Part model, mm, in its own coordinate system. Face numbers are marked on the shaded views. A direction names the side the tool comes from. Coordinates: 2 decimals unless noted, no trailing zeros. Write each loop counter-clockwise with the first axis right and the second up, starting at its lowest first coordinate (ties: lowest second). Pieces come first, ordered by that corner, then holes. Notation, with made-up numbers: (25, -21.75) - (29, -21.75) arc R14 cw to (29, -17.75) - close; hole circle Ø11 at (37, 7). An arc over 180 degrees is marked (long way). Use a Markdown table: item, result.
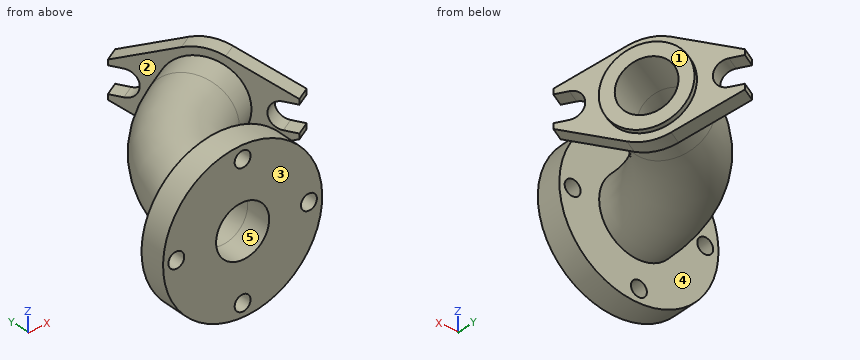
```python
from build123d import *

# Parameters (mm, degrees)
SKETCH_1_R      = 30
SKETCH_1_R_2    = 10
SKETCH_1_R_3    = 3
EXTRUDE_1_DEPTH = 10
SKETCH_2_R      = 15
SKETCH_2_R_2    = 10
EXTRUDE_START   = -6
SKETCH_5_R      = 10
EXTRUDE_2_DEPTH = 6


with BuildPart() as part:
    # 草图1 → 凸台-拉伸1 (new body)
    with BuildSketch(Plane(origin=(0, 0, 0), x_dir=(1, 0, 0), z_dir=(0, 1, 0))):
        with Locations(Location((0, 0, 0), (0, 0, 270))):
            Circle(SKETCH_1_R)
        with Locations(Location((0, 0, 0), (0, 0, 270))):
            Circle(SKETCH_1_R_2, mode=Mode.SUBTRACT)
        with Locations(Location((25, 0, 0), (0, 0, 270))):
            Circle(SKETCH_1_R_3, mode=Mode.SUBTRACT)
        with Locations(Location((0, -25, 0), (0, 0, 270))):
            Circle(SKETCH_1_R_3, mode=Mode.SUBTRACT)
        with Locations(Location((-25, 0, 0), (0, 0, 270))):
            Circle(SKETCH_1_R_3, mode=Mode.SUBTRACT)
        with Locations(Location((0, 25, 0), (0, 0, 270))):
            Circle(SKETCH_1_R_3, mode=Mode.SUBTRACT)
    extrude(amount=EXTRUDE_1_DEPTH)

    # 扫描1: sweep along a path in 草图3
    with BuildLine(Plane.XY) as sweep_1_path:
        Line((43.088457268, 66.631397208), (27.5, 57.631397208))
        ThreePointArc((27.5, 57.631397208), (7.368602792, 37.5), (0, 10))
    # 草图2 → 扫描1 (sweep)
    with BuildSketch(Plane(origin=(0, 10, 0), x_dir=(1, 0, 0), z_dir=(0, 1, 0))):
        Circle(SKETCH_2_R)
        Circle(SKETCH_2_R_2, mode=Mode.SUBTRACT)
    sweep(path=sweep_1_path.line)

    # 草图5 → 凸台-拉伸2 (add)
    with BuildSketch(Plane(origin=(59.436533479, 34.315698604, 0), x_dir=(0, 0, -1), z_dir=(0.866025403784436, 0.5000000000000044, 0)).offset(EXTRUDE_START)):
        with BuildLine():
            Line((-7, 6.160254038), (-5, 6.160254038))
            Line((-5, 6.160254038), (-5, 11.160254038))
            ThreePointArc((-5, 11.160254038), (0, 16.160254038), (5, 11.160254038))
            Line((5, 11.160254038), (5, 6.160254038))
            Line((5, 6.160254038), (7, 6.160254038))
            Line((7, 6.160254038), (16.615384615, 29.237177115))
            ThreePointArc((16.615384615, 29.237177115), (18, 36.160254038), (16.615384615, 43.083330961))
            Line((16.615384615, 43.083330961), (7, 66.160254038))
            Line((7, 66.160254038), (5, 66.160254038))
            Line((5, 66.160254038), (5, 61.160254038))
            ThreePointArc((5, 61.160254038), (0, 56.160254038), (-5, 61.160254038))
            Line((-5, 61.160254038), (-5, 66.160254038))
            Line((-5, 66.160254038), (-7, 66.160254038))
            Line((-7, 66.160254038), (-16.615384615, 43.083330961))
            ThreePointArc((-16.615384615, 43.083330961), (-18, 36.160254038), (-16.615384615, 29.237177115))
            Line((-16.615384615, 29.237177115), (-7, 6.160254038))
        make_face()
        with Locations(Location((0, 36.160254038, 0), (0, 0, 90))):
            Circle(SKETCH_5_R, mode=Mode.SUBTRACT)
    extrude(amount=EXTRUDE_2_DEPTH)


solid = part.part
```
Item 1: Two-plate mould, pull along X, no slides. Class the marked faces 1, 2 and 3: pulls with the +X half, pulls with the -X half, needs draft (parallel to the pull), parting line crosses it, or undercut.
From the geometry:
| item | result |
|---|---|
| face 1 | pulls with the +X half |
| face 2 | undercut |
| face 3 | needs draft |
Item 2: Band-saw the part on C-C, the plane x = -25. Give the cut face in (y, z), then the cut area to 3 significant figures.
From the geometry:
| item | result |
|---|---|
| outline | (0, -16.58) - (10, -16.58) - (10, -3) - (0, -3) - close; (0, 3) - (10, 3) - (10, 16.58) - (0, 16.58) - close |
| area | 272 mm^2 |
Item 3: Band-saw the part on A-A, the plane z = -25. Give the cut face in (x, y), then the cut area to 3 significant figures.
From the geometry:
| item | result |
|---|---|
| outline | (-16.58, 0) - (-3, 0) - (-3, 10) - (-16.58, 10) - close; (3, 0) - (16.58, 0) - (16.58, 10) - (3, 10) - close |
| area | 272 mm^2 |
Item 4: Band-saw the part on B-B, the plane z = 0. Count the separate pieces of the cut face and the enclosed holes in it, then the cut area to 3 significant figures.
From the geometry:
| item | result |
|---|---|
| separate pieces | 4 |
| enclosed holes | 0 |
| area | 1,100 mm^2 |
Item 5: Drill centre lines: probe 1 along X at (y, z) = (7, 0); probe 2 along X at (y, z) = (45, -6.5); probe 3 along Y at (x, z) = (-25, -12.5). Where is each one in solid material? Low to high.
From the geometry:
| item | result |
|---|---|
| probe 1 | -30 to -28, -22 to -10, 10 to 22, 28 to 30 |
| probe 2 | -3.9 to 3.1, 23.03 to 32.74, 46.34 to 53.27 |
| probe 3 | 0 to 10 |
Item 6: Which spindle directions (+Z, -Z, +X, -X, +Y, -Y) get a long thin tool onto all of the face, cutting with end or side? Do the marked faces 4 and 5. Say none if no direction does.
From the geometry:
| item | result |
|---|---|
| face 4 | none |
| face 5 | -Y |
Item 7: Drop flat-ended pins along their axis: P1, Ø5.5, axis at x = 25, z = 0, coming from the +Y side; P2, Ø4, axis at x = -10, z = 12, coming from the -Y side; P3, Ø3.5, axis at x = 52, y = 39, coming from the +Z side; P4, Ø2, axis at x = 24.5, y = 71.5, coming from the +Z side. Give the stop position or say it passes through.
From the geometry:
| item | result |
|---|---|
| P1 | y = 80.88 |
| P2 | y = 0 |
| P3 | z = 8.4 |
| P4 | z = 8.28 |
